Here's the drawing with two shaded views (mm, measured from the low corner). I have some questions. Coordinates: 2 decimals unless noted, no trailing zeros. Write each loop counter-clockwise with the first axis right and the second up, starting at its lowest first coordinate (ties: lowest second). Pieces come first, ordered by that corner, then holes.
Item 1: If we section it at B-B (z = 22.5): Please give me the cut outline in (x, y), then the cut area to 3 significant figures.
Item 2: If we section it at A-A (x = 36): Please give me the cut outline in (y, z).
Item 3: If I drill on line 1 (Z direction, x = 102.5, y = 1.2); line 2 (Z direction, x = 112, y = 1.15); line 3 (Z direction, x = 77, y = 1.9), over which ranges is the centre line in solid material (lowest first)?
Item 4: If we section it at C-C (y = 0.75): Please give me the cut outline in (x, z), then the cut area to 3 significant figures.
Item 5: I'm going to push flat-ended pins straight in: pin 1 Ø0.6 at (x, y) = (61.5, 1.5) entering from -Z; pin 2 Ø12 at (x, z) = (81.5, 21) entering from +Y. Where does each tip first touch, or does it pass through?
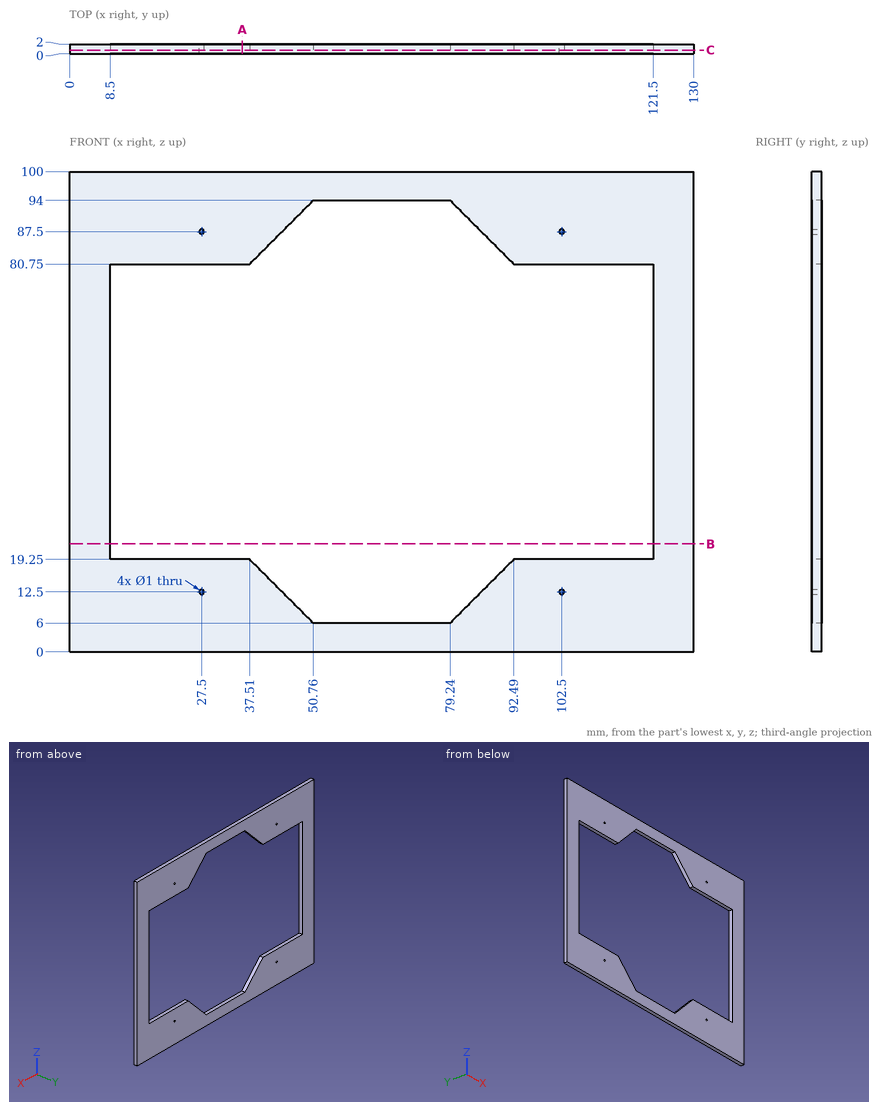
Answer list:
1. outline: (0, 0) - (8.5, 0) - (8.5, 2) - (0, 2) - close; (121.5, 0) - (130, 0) - (130, 2) - (121.5, 2) - close
1. area: 34.0 mm2
2. outline: (0, 0) - (2, 0) - (2, 19.25) - (0, 19.25) - close; (0, 80.75) - (2, 80.75) - (2, 100) - (0, 100) - close
3. line 1: z = 0 to 12, 13 to 19.25, 80.75 to 87, 88 to 100
3. line 2: z = 0 to 19.25, 80.75 to 100
3. line 3: z = 0 to 6, 94 to 100
4. outline: (0, 0) - (130, 0) - (130, 100) - (0, 100) - close; hole (8.5, 19.25) - (37.51, 19.25) - (50.76, 6) - (79.24, 6) - (92.49, 19.25) - (121.5, 19.25) - (121.5, 80.75) - (92.49, 80.75) - (79.24, 94) - (50.76, 94) - (37.51, 80.75) - (8.5, 80.75) - close; hole circle Ø1 at (27.5, 12.5); hole circle Ø1 at (27.5, 87.5); hole circle Ø1 at (102.5, 12.5); hole circle Ø1 at (102.5, 87.5)
4. area: 4,940 mm2
5. pin 1: stops at z = 0
5. pin 2: passes through
